Check sheet for the drawn part. Datum: minimum x, y, z corner. Units: mm. A direction names the side the tool comes from. Round coordinates to 2 decimals unless told otherwise and drop trailing zeros. Order: outer loops, then holes, each group sorted by start corner. A loop starts at its lowest first (then second) coordinate and runs counter-clockwise, first axis right, second up.
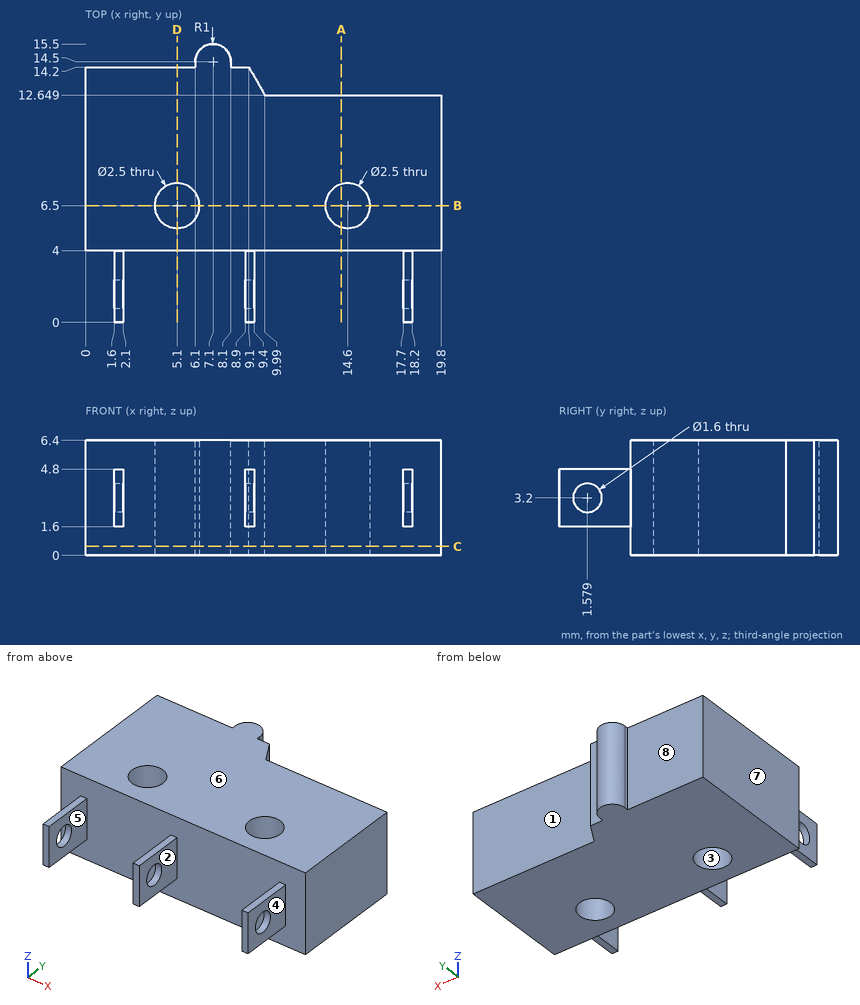
(1) Sectioned sample at D-D, the plane x = 5.1. Record the cut outline in (y, z).
Returned:
outline: (4, 0) - (5.25, 0) - (5.25, 6.4) - (4, 6.4) - close; (7.75, 0) - (14.2, 0) - (14.2, 6.4) - (7.75, 6.4) - close
(2) Material ranges on line 1 (Y direction, x = 14.6, z = 3.75); line 2 (Y direction, x = 5.1, z = 4.25); line 3 (Y direction, x = 16, z = 2.5), recorded low to high.
Returned:
line 1: y = 4 to 5.25, 7.75 to 12.65
line 2: y = 4 to 5.25, 7.75 to 14.2
line 3: y = 4 to 12.65
(3) Draft check along Y on the marked faces 1, 2 and 3. Enter one of: released by +Y, released by -Y, zero draft, split by the parting line, or undercut.
Returned:
face 1: released by +Y
face 2: zero draft
face 3: undercut
(4) Depth check by flat-ended pin: P1, Ø1.4, axis at y = 1.58, z = 3.2, coming from the -X side; P2, Ø0.6, axis at x = 2, y = 1.5, coming from the -Z side; P3, Ø3, axis at x = 15.5, z = 2, coming from the +Y side; P4, Ø1.6, axis at y = 1.5, z = 2.5, coming from the +X side. Enter the tip coordinate at first touch or a pass-through.
Returned:
P1: passes through
P2: stops at z = 1.6
P3: stops at y = 12.65
P4: stops at x = 18.2
(5) Set-up check for the marked faces 4, 5, 6, 7 and 8: record each of +Z, -Z, +X, -X, +Y, -Y from which the full face is reachable in a straight line by a thin tool's end or side.
Returned:
face 4: +Z, -Z, +X, -Y
face 5: +Z, -Z, -Y
face 6: +Z, +X, -X, +Y, -Y
face 7: +Z, -Z, -X, +Y, -Y
face 8: +Z, -Z, -X, +Y
(6) Sectioned sample at B-B, the plane y = 6.5. Record the cut outline in (x, z).
Returned:
outline: (0, 0) - (3.85, 0) - (3.85, 6.4) - (0, 6.4) - close; (6.35, 0) - (13.35, 0) - (13.35, 6.4) - (6.35, 6.4) - close; (15.85, 0) - (19.8, 0) - (19.8, 6.4) - (15.85, 6.4) - close
(7) Sectioned sample at C-C, the plane z = 0.5. Record the cut outline in (x, y).
Returned:
outline: (0, 4) - (19.8, 4) - (19.8, 12.65) - (9.99, 12.65) - (9.1, 14.2) - (8.1, 14.2) - (8.1, 14.5) arc R1 ccw (long way) to (6.1, 14.49) - (6.1, 14.2) - (0, 14.2) - close; hole circle Ø2.5 at (5.1, 6.5); hole circle Ø2.5 at (14.6, 6.5)
(8) Sectioned sample at A-A, the plane x = 14.25. Record the cut outline in (y, z).
Returned:
outline: (4, 0) - (5.3, 0) - (5.3, 6.4) - (4, 6.4) - close; (7.7, 0) - (12.65, 0) - (12.65, 6.4) - (7.7, 6.4) - close
